Read the model definition and answer for the solid it produces. Units are mm, in the model's axes. A direction names the side the tool comes from. Round coordinates to 2 decimals unless told otherwise and drop trailing zeros. Write each loop counter-clockwise with the first axis right and the second up, starting at its lowest first coordinate (ties: lowest second). Pieces come first, ordered by that corner, then holes. Notation, with made-up numbers: (66, 72.5) -> (75, 72.5) arc R17 ccw to (75, 98.5) -> close; hole circle Ø11 at (-40, -28). An arc over 180 degrees is marked (long way). Return JSON: item names as keys, results as strings. Group by question number.
(1) The mould has two halves that part along Y. Classify faces 1 (the flat face through (10, 0, 25.9)), 2 (the flat face through (3.4, -3.4, 28.4)): released by +Y, released by -Y, zero draft, split by the parting line, or undercut.
(2) Given pin 1 (0.9 mm diameter, centred on x = 0.5, y = -10.5, fed in from +Z); pin 2 (2 mm diameter, centred on x = -13.5, z = 16.5, fed in from -Y); pin 3 (2 mm diameter, centred on x = 11, z = 12.5, fed in from +Y), each flat-ended and moving along its own axis, determine where each tip first touches the part or whether it passes through.
(3) For faces 3 (the cylindrical face through (-0.325, 8.536, 27.132)), 4 (the flat face through (-8, 13, 3)), 5 (the cylindrical face through (-0.59, 4.46, 14.4)), determine the directions among +Z, -Z, +X, -X, +Y, -Y from which every point of the face is accessible in a straight line to the end or side of a thin tool.
(4) A cutting plane is placed at A-A on z = 23. Give the vertices of the cut face in (x, y).
(5) Straight lines are drawn through the part: line 1 (Y direction, x = 0, z = 26.4); line 2 (Y direction, x = -1.5, z = 9.25); line 3 (X direction, y = -10, z = 27). For each, find the intervals that lie inside material, in ascending order.
```python
from build123d import *

# Parameters (mm, degrees)
ESQUISSE1_R             = 17.25
BOSS_EXTRU_1_DEPTH      = 28.4
CHANFREIN1_SIZE         = 1
ESQUISSE2_R             = 1.5
ESQUISSE2_R_2           = 1.25
ENL_V_MAT_EXTRU_1_DEPTH = 3
ENL_V_START             = -2.5
ESQUISSE3_R             = 1.5
ENL_V_MAT_EXTRU_2_DEPTH = 2.5
ESQUISSE4_R             = 4.5
ENL_V_MAT_EXTRU_4_DEPTH = 38.439083856


with BuildPart() as part:
    # Esquisse1 → Boss.-Extru.1 (new body)
    with BuildSketch(Plane.XY):
        Circle(ESQUISSE1_R)
    extrude(amount=BOSS_EXTRU_1_DEPTH)

    # Chanfrein1
    chanfrein1_edges = [part.edges().sort_by_distance(p)[0] for p in [
        (-17.25, 0, 28.4),
    ]]
    chamfer(chanfrein1_edges, length=CHANFREIN1_SIZE)

    # Esquisse2 → Enlèv. mat.-Extru.1 (cut)
    with BuildSketch(Plane(origin=(0, 0, 0), x_dir=(-1, 0, 0), z_dir=(0, 0, -1))):
        with Locations((8.660254038, 5)):
            Circle(ESQUISSE2_R)
        with Locations((0, -10)):
            Circle(ESQUISSE2_R)
        with Locations((-8.660254038, 5)):
            Circle(ESQUISSE2_R)
        with Locations((7.713223432, 13.359694875)):
            Circle(ESQUISSE2_R_2)
        with Locations((7.713223432, -13.359694875)):
            Circle(ESQUISSE2_R_2)
        with Locations((-15.426446864, 0)):
            Circle(ESQUISSE2_R_2)
    extrude(amount=-ENL_V_MAT_EXTRU_1_DEPTH, mode=Mode.SUBTRACT)

    # Esquisse3 → Enlèv. mat.-Extru.2 (cut)
    with BuildSketch(Plane.XY.offset(28.4).offset(ENL_V_START)):
        with Locations((0, 10)):
            Circle(ESQUISSE3_R)
        with Locations((10, 0)):
            Circle(ESQUISSE3_R)
        with Locations(Location((0, -10, 0), (0, 0, 180))):
            Circle(ESQUISSE3_R)
        with Locations((-10, 0)):
            Circle(ESQUISSE3_R)
    extrude(amount=ENL_V_MAT_EXTRU_2_DEPTH, mode=Mode.SUBTRACT)

    # Esquisse4 → Enlèv. mat.-Extru.4 (cut, through all)
    with BuildSketch(Plane.XY.offset(28.4)):
        Circle(ESQUISSE4_R)
    extrude(amount=-ENL_V_MAT_EXTRU_4_DEPTH, mode=Mode.SUBTRACT)


solid = part.part
```
Checks:
{
 "1": {"face 1": "undercut", "face 2": "zero draft"},
 "2": {"pin 1": "stops at z = 25.9", "pin 2": "stops at y = -11.89", "pin 3": "stops at y = 14.06"},
 "3": {"face 3": "+Z", "face 4": "-Z", "face 5": "+Z, -Z"},
 "4": {"outline": "circle Ø34.5 at (0, 0); hole circle Ø9 at (0, 0)"},
 "5": {"line 1": "y = -17.25 to -11.5, -8.5 to -4.5, 4.5 to 8.5, 11.5 to 17.25", "line 2": "y = -17.18 to -4.24, 4.24 to 17.18", "line 3": "x = -14.06 to -1.5, 1.5 to 14.06"}
}
